Geometry check sheet. Reference: the model listing, model coordinates, mm. A direction names the side the tool comes from. Give positions to 0.01 mm unless a question says otherwise; leave off trailing zeros. Write each loop counter-clockwise with the first axis right and the second up, starting at its lowest first coordinate (ties: lowest second). Pieces come first, ordered by that corner, then holes. Notation, with made-up numbers: M 44,69 L 55,69 A22 ccw 55,76 Z; hole C 74,44 d11. An arc over 180 degrees is marked long. Write each question's results on one line, items separated by ' | '.
```python
from build123d import *

# Parameters (mm, degrees)
F1_DEPTH = 2.667
F2_R     = 6.985
F3_DEPTH = 1.524
F5_DEPTH = 0.8255
F7_DEPTH = 2.668


with BuildPart() as f1:
    # F0 (on Top) → F1 (new body)
    with BuildSketch(Plane.XY):
        with BuildLine():
            Line((215.9, 171.45), (-215.9, 171.45))
            Line((-215.9, 171.45), (-215.9, -142.875))
            ThreePointArc((-215.9, -142.875), (-216.829936, -145.120064), (-219.075, -146.05))
            Line((-219.075, -146.05), (-241.3, -146.05))
            Line((-241.3, -146.05), (-241.3, -171.45))
            Line((-241.3, -171.45), (215.9, -171.45))
            Line((215.9, -171.45), (215.9, 171.45))
        make_face()
    extrude(amount=F1_DEPTH)

    # F2 (on face) → F3 (cut)
    with BuildSketch(Plane(origin=(0, 0, 0), x_dir=(1, 0, 0), z_dir=(0, 0, -1))):
        with Locations((-196.85, 163.195)):
            Circle(F2_R)
        with Locations((120.65, 163.195)):
            Circle(F2_R)
    extrude(amount=-F3_DEPTH, mode=Mode.SUBTRACT)

    # F4 (on face) → F5 (cut)
    with BuildSketch(Plane.XY.offset(2.667)):
        with BuildLine():
            Line((-81.065625, -39.87), (81.065625, -39.87))
            ThreePointArc((81.065625, -39.87), (91.905753, -44.360128), (87.415625, -33.52))
            Line((87.415625, -33.52), (87.415625, 33.52))
            ThreePointArc((87.415625, 33.52), (91.905753, 44.360128), (81.065625, 39.87))
            Line((81.065625, 39.87), (-81.065625, 39.87))
            ThreePointArc((-81.065625, 39.87), (-91.905753, 44.360128), (-87.415625, 33.52))
            Line((-87.415625, 33.52), (-87.415625, -33.52))
            ThreePointArc((-87.415625, -33.52), (-91.905753, -44.360128), (-81.065625, -39.87))
        make_face()
        with BuildLine():
            Line((-80.430625, 36.06), (80.430625, 36.06))
            ThreePointArc((80.430625, 36.06), (82.675689, 35.130064), (83.605625, 32.885))
            Line((83.605625, 32.885), (83.605625, -32.885))
            ThreePointArc((83.605625, -32.885), (82.675689, -35.130064), (80.430625, -36.06))
            Line((80.430625, -36.06), (-80.430625, -36.06))
            ThreePointArc((-80.430625, -36.06), (-82.675689, -35.130064), (-83.605625, -32.885))
            Line((-83.605625, -32.885), (-83.605625, 32.885))
            ThreePointArc((-83.605625, 32.885), (-82.675689, 35.130064), (-80.430625, 36.06))
        make_face(mode=Mode.SUBTRACT)
    extrude(amount=-F5_DEPTH, mode=Mode.SUBTRACT)

    # F6 (on face) → F7 (cut, through all)
    with BuildSketch(Plane.XY.offset(2.667)):
        with BuildLine():
            Line((83.605625, -32.885), (83.605625, 32.885))
            ThreePointArc((83.605625, 32.885), (82.675689, 35.130064), (80.430625, 36.06))
            Line((80.430625, 36.06), (-80.430625, 36.06))
            ThreePointArc((-80.430625, 36.06), (-82.675689, 35.130064), (-83.605625, 32.885))
            Line((-83.605625, 32.885), (-83.605625, -32.885))
            ThreePointArc((-83.605625, -32.885), (-82.675689, -35.130064), (-80.430625, -36.06))
            Line((-80.430625, -36.06), (80.430625, -36.06))
            ThreePointArc((80.430625, -36.06), (82.675689, -35.130064), (83.605625, -32.885))
        make_face()
    extrude(amount=-F7_DEPTH, mode=Mode.SUBTRACT)


solid = f1.part
```
Q1. Section check C-C (x = 120.65). Enter the section's corners in (y, z).
Answer key:
outline: M -171.45,0 L -170.18,0 L -170.18,1.52 L -156.21,1.52 L -156.21,0 L 171.45,0 L 171.45,2.67 L -171.45,2.67 Z
Q2. Section check D-D (z = 0.75). Enter the section's corners in (x, y) (3 decimals), then the cut area to 3 significant figures.
Answer key:
outline: M -241.3,-171.45 L 215.9,-171.45 L 215.9,171.45 L -215.9,171.45 L -215.9,-142.875 A3.175 cw -219.075,-146.05 L -241.3,-146.05 Z; hole C -196.85,-163.195 d13.97; hole M -83.606,-32.885 A3.175 ccw -80.431,-36.06 L 80.431,-36.06 A3.175 ccw 83.606,-32.885 L 83.606,32.885 A3.175 ccw 80.431,36.06 L -80.431,36.06 A3.175 ccw -83.606,32.885 Z; hole C 120.65,-163.195 d13.97 | area: 136,000 mm2
Q3. Depth check by flat-ended pin: P1, Ø0.8, axis at y = 61, z = 2, coming from the -X side; P2, Ø10, axis at x = 87.42, y = 39.87, coming from the +Z side; P3, Ø4, axis at x = 118, y = -165.5, coming from the -Z side. Enter the tip coordinate at first touch or a pass-through.
Answer key:
P1: stops at x = -215.9 | P2: stops at z = 1.84 | P3: stops at z = 1.52
Q4. Section check B-B (y = 11). Enter the section's corners in (x, z), then the cut area to 3 significant figures.
Answer key:
outline: M -215.9,0 L -83.61,0 L -83.61,1.84 L -87.42,1.84 L -87.42,2.67 L -215.9,2.67 Z; M 83.61,0 L 215.9,0 L 215.9,2.67 L 87.42,2.67 L 87.42,1.84 L 83.61,1.84 Z | area: 699 mm2
Q5. Access from +Z, -Z, +X, -X, +Y, -Y to the whole of each face (thin tool, end or side, straight path). Record for faces 4 (the face through (-16, 41, 2.667)), 5 (the face through (-92.05, -44.21, 2.26)), 6 (the face through (-197, -163, 1.524)).
Answer key:
face 4: +Z, +X, -X, +Y, -Y | face 5: +Z | face 6: -Z
Q6. Release check for a two-part mould opening along Y. For faces 1 (the face through (-21, -37, 1.842)), 2 (the face through (-16, 41, 0)), 3 (the face through (91.755, -44.506, 2.26)) record: released by +Y, released by -Y, zero draft, split by the parting line, or undercut.
Answer key:
face 1: undercut | face 2: zero draft | face 3: undercut
Q7. Section check A-A (x = -5). Enter the section's corners in (y, z).
Answer key:
outline: M -171.45,0 L -36.06,0 L -36.06,1.84 L -39.87,1.84 L -39.87,2.67 L -171.45,2.67 Z; M 36.06,0 L 171.45,0 L 171.45,2.67 L 39.87,2.67 L 39.87,1.84 L 36.06,1.84 Z
Q8. Material ranges on probe 1 along X at (y, z) = (-33, 0.6); probe 2 along Y at (x, z) = (38.5, 2.15); probe 3 along Y at (x, z) = (-196.85, 0.65), recorded low to high. Write a range as [from, to].
Answer key:
probe 1: x = [-215.9, -83.6], [83.6, 215.9] | probe 2: y = [-171.45, -39.87], [39.87, 171.45] | probe 3: y = [-171.45, -170.18], [-156.21, 171.45]
